```python
from build123d import *

# Parameters (mm, degrees)
F0_R     = 1.6
F1_DEPTH = 3.175


with BuildPart() as f1:
    # F0 (on Front) → F1 (new body)
    with BuildSketch(Plane.XZ):
        with BuildLine():
            Line((63.081035, 75.419807), (-34.218965, 75.419807))
            ThreePointArc((-34.218965, 75.419807), (-38.709093, 73.559935), (-40.568965, 69.069807))
            Line((-40.568965, 69.069807), (-40.568965, -68.230193))
            ThreePointArc((-40.568965, -68.230193), (-38.709093, -72.720321), (-34.218965, -74.580193))
            Line((-34.218965, -74.580193), (63.081035, -74.580193))
            ThreePointArc((63.081035, -74.580193), (67.571163, -72.720321), (69.431035, -68.230193))
            Line((69.431035, -68.230193), (69.431035, 69.069807))
            ThreePointArc((69.431035, 69.069807), (67.571163, 73.559935), (63.081035, 75.419807))
        make_face()
        with Locations((-35.568965, -69.560093)):
            Circle(F0_R, mode=Mode.SUBTRACT)
        with Locations((-35.568965, -59.560093)):
            Circle(F0_R, mode=Mode.SUBTRACT)
        with Locations((-25.568965, -69.539993)):
            Circle(F0_R, mode=Mode.SUBTRACT)
        with Locations((-15.568965, -69.539993)):
            Circle(F0_R, mode=Mode.SUBTRACT)
        with Locations((-35.568965, -49.560093)):
            Circle(F0_R, mode=Mode.SUBTRACT)
        with Locations((-35.568965, -39.560093)):
            Circle(F0_R, mode=Mode.SUBTRACT)
        with Locations((-5.568965, -69.539993)):
            Circle(F0_R, mode=Mode.SUBTRACT)
        with Locations((4.431035, -69.539993)):
            Circle(F0_R, mode=Mode.SUBTRACT)
        with Locations((14.431035, -69.539993)):
            Circle(F0_R, mode=Mode.SUBTRACT)
        with Locations((-35.568965, -29.560093)):
            Circle(F0_R, mode=Mode.SUBTRACT)
        with Locations((-35.568965, -19.560093)):
            Circle(F0_R, mode=Mode.SUBTRACT)
        with Locations((-35.568965, -9.560093)):
            Circle(F0_R, mode=Mode.SUBTRACT)
        with Locations((24.431035, -69.539993)):
            Circle(F0_R, mode=Mode.SUBTRACT)
        with Locations((34.431035, -69.539993)):
            Circle(F0_R, mode=Mode.SUBTRACT)
        with Locations((44.431035, -69.539993)):
            Circle(F0_R, mode=Mode.SUBTRACT)
        with Locations((54.431035, -69.539993)):
            Circle(F0_R, mode=Mode.SUBTRACT)
        with Locations((64.431035, -69.560093)):
            Circle(F0_R, mode=Mode.SUBTRACT)
        with Locations((64.431035, -59.560093)):
            Circle(F0_R, mode=Mode.SUBTRACT)
        with Locations((64.431035, -49.560093)):
            Circle(F0_R, mode=Mode.SUBTRACT)
        with Locations((64.431035, -39.560093)):
            Circle(F0_R, mode=Mode.SUBTRACT)
        with Locations((64.431035, -29.560093)):
            Circle(F0_R, mode=Mode.SUBTRACT)
        with Locations((64.431035, -19.560093)):
            Circle(F0_R, mode=Mode.SUBTRACT)
        with Locations((64.431035, -9.560093)):
            Circle(F0_R, mode=Mode.SUBTRACT)
        with Locations((-35.568965, 0.439907)):
            Circle(F0_R, mode=Mode.SUBTRACT)
        with Locations((-35.568965, 10.439907)):
            Circle(F0_R, mode=Mode.SUBTRACT)
        with Locations((-35.568965, 20.439907)):
            Circle(F0_R, mode=Mode.SUBTRACT)
        with Locations((-35.568965, 30.439907)):
            Circle(F0_R, mode=Mode.SUBTRACT)
        with Locations((-35.568965, 40.439907)):
            Circle(F0_R, mode=Mode.SUBTRACT)
        with Locations((-35.568965, 50.439907)):
            Circle(F0_R, mode=Mode.SUBTRACT)
        with Locations((-35.568965, 60.439907)):
            Circle(F0_R, mode=Mode.SUBTRACT)
        with Locations((-35.568965, 70.439907)):
            Circle(F0_R, mode=Mode.SUBTRACT)
        with Locations((-25.568965, 70.419807)):
            Circle(F0_R, mode=Mode.SUBTRACT)
        with Locations((-15.568965, 70.419807)):
            Circle(F0_R, mode=Mode.SUBTRACT)
        with Locations((-5.568965, 70.419807)):
            Circle(F0_R, mode=Mode.SUBTRACT)
        with Locations((4.431035, 70.419807)):
            Circle(F0_R, mode=Mode.SUBTRACT)
        with Locations((14.431035, 70.419807)):
            Circle(F0_R, mode=Mode.SUBTRACT)
        with BuildLine():
            ThreePointArc((-22.913965, 55.899907), (-21.054093, 60.390035), (-16.563965, 62.249907))
            Line((-16.563965, 62.249907), (45.426035, 62.249907))
            ThreePointArc((45.426035, 62.249907), (49.916163, 60.390035), (51.776035, 55.899907))
            Line((51.776035, 55.899907), (51.776035, -55.020093))
            ThreePointArc((51.776035, -55.020093), (49.916163, -59.510221), (45.426035, -61.370093))
            Line((45.426035, -61.370093), (-16.563965, -61.370093))
            ThreePointArc((-16.563965, -61.370093), (-21.054093, -59.510221), (-22.913965, -55.020093))
            Line((-22.913965, -55.020093), (-22.913965, 55.899907))
        make_face(mode=Mode.SUBTRACT)
        with Locations((64.431035, 0.439907)):
            Circle(F0_R, mode=Mode.SUBTRACT)
        with Locations((64.431035, 10.439907)):
            Circle(F0_R, mode=Mode.SUBTRACT)
        with Locations((64.431035, 20.439907)):
            Circle(F0_R, mode=Mode.SUBTRACT)
        with Locations((64.431035, 30.439907)):
            Circle(F0_R, mode=Mode.SUBTRACT)
        with Locations((24.431035, 70.419807)):
            Circle(F0_R, mode=Mode.SUBTRACT)
        with Locations((34.431035, 70.419807)):
            Circle(F0_R, mode=Mode.SUBTRACT)
        with Locations((64.431035, 40.439907)):
            Circle(F0_R, mode=Mode.SUBTRACT)
        with Locations((64.431035, 50.439907)):
            Circle(F0_R, mode=Mode.SUBTRACT)
        with Locations((44.431035, 70.419807)):
            Circle(F0_R, mode=Mode.SUBTRACT)
        with Locations((54.431035, 70.419807)):
            Circle(F0_R, mode=Mode.SUBTRACT)
        with Locations((64.431035, 60.439907)):
            Circle(F0_R, mode=Mode.SUBTRACT)
        with Locations((64.431035, 70.439907)):
            Circle(F0_R, mode=Mode.SUBTRACT)
    extrude(amount=F1_DEPTH)


solid = f1.part
```
The listing builds one solid part. Answer for the finished solid, in the listing's coordinates (mm). A direction names the side the tool comes from. Coordinates: 2 decimals unless noted, no trailing zeros. Write each loop counter-clockwise with the first axis right and the second up, starting at its lowest first coordinate (ties: lowest second). Pieces come first, ordered by that corner, then holes. Notation, with made-up numbers: M 36,-27.5 L 93,-27.5 A15 cw 93,-16.5 Z; hole C 38,-2.75 d3. An arc over 180 degrees is marked long. Use a Markdown table: item, result. Add a question column.
1. Straight lines are drawn through the part: line 1 along X through (y, z) = (-1.05, 24.5); line 2 along Z through (x, y) = (10, -2.35); line 3 along X through (y, z) = (-0.25, -28.5). For each, find the intervals that lie inside material, in ascending order. Write a range as [from, to].
2. Section A-A (z = -43) is taken. Give the vertices of the cut face in (x, y) (3 decimals), plus the area to 3 significant figures.
3. Section C-C (y = -0.85) is taken. Count the separate pieces of the cut face and the enclosed holes in it, plus the area to 3 significant figures.
4. Section B-B (x = 9) is taken. Give the vertices of the cut face in (y, z) (3 decimals), plus the area to 3 significant figures.
5. For a pull along Z with two mould halves and no side action, classify faces 1 (the flat face through (-35, -3.175, 18)), 2 (the flat face through (14, -2, -74.58)), 3 (the cylindrical face through (-24.71, -1.57, 71.77)), 4 (the cylindrical face through (-38.66, -1.57, 73.61)) as +Z half, -Z half, draft (parallel to the pull), parting line (faces both ways), or undercut.
6. Which of the six approach directions +Z, -Z, +X, -X, +Y, -Y give full straight-line access (tool end or side, diameter ignored) to faces 5 (the flat face through (-40.569, -2, 1)), 6 (the flat face through (14, -2, 62.25))?
Data:
| question | item | result |
|---|---|---|
| 1 | line 1 | x = [-40.57, -22.91], [51.78, 69.43] |
| 1 | line 2 | z = [-74.58, -61.37], [62.25, 75.42] |
| 1 | line 3 | x = [-40.57, -36.77], [-34.37, -22.91], [51.78, 63.23], [65.63, 69.43] |
| 2 | outline | M -40.569,-3.175 L -22.914,-3.175 L -22.914,0 L -40.569,0 Z; M 51.776,-3.175 L 69.431,-3.175 L 69.431,0 L 51.776,0 Z |
| 2 | area | 112 mm2 |
| 3 | separate pieces | 1 |
| 3 | enclosed holes | 49 |
| 3 | area | 6,880 mm2 |
| 4 | outline | M -3.175,-74.58 L 0,-74.58 L 0,-61.37 L -3.175,-61.37 Z; M -3.175,62.25 L 0,62.25 L 0,75.42 L -3.175,75.42 Z |
| 4 | area | 83.8 mm2 |
| 5 | face 1 | draft |
| 5 | face 2 | -Z half |
| 5 | face 3 | undercut |
| 5 | face 4 | +Z half |
| 6 | face 5 | +Z, -Z, -X, +Y, -Y |
| 6 | face 6 | +Y, -Y |
